Source: CAD feature listing. Evaluate the final solid. Frame: model axes, mm. A direction names the side the tool comes from. Give positions to 0.01 mm unless a question says otherwise; leave off trailing zeros. Order: outer loops, then holes, each group sorted by start corner. A loop starts at its lowest first (then second) coordinate and runs counter-clockwise, first axis right, second up. Notation, with made-up numbers: M -1,69 L 39,69 A14 ccw 39,76 Z; hole C 84,-11.5 d11. An arc over 180 degrees is marked long. Answer in a Markdown table with one row per item. Add a question column.
(1) Set-up query: faces 1 (the face through (-14.985, 0.66, 12.028)), 2 (the face through (4, 4, 4)), 3 (the face through (0, -2, 5)). Return all of +Z, -Z, +X, -X, +Y, -Y with unobstructed straight access to the full face (end or side cutting, diameter ignored); none if empty.
(2) Section query D-D, the plane y = 6. Return loops of the section in (x, z), plus the area to 3 significant figures.
(3) Mould query, pull axis Y, two halves, no side actions, for faces 4 (the face through (14.985, 0.66, 1.972)), 5 (the face through (2.2, 0.1, 0)), 6 (the face through (20.03, 6.31, 6.9)). Classes: pulls with the +Y half, pulls with the -Y half, needs draft (parallel to the pull), parting line crosses it, or undercut.
(4) Section query B-B, the plane y = 0. Return loops of the section in (x, z).
(5) Pin query (flat end, axial travel): P1, Ø3.5, axis at x = -10.39, y = -6, coming from the -Z side; P2, Ø5, axis at x = 16.5, z = 9.5, coming from the -Y side; P3, Ø4.5, axis at x = 10.39, y = -6, coming from the -Z side; P4, Ø8, axis at x = 11, z = 12, coming from the -Y side. Return the tip coordinate at first contact, or that it passes through.
(6) Section query A-A, the plane x = 0. Return loops of the section in (y, z).
(7) Material intervals for line 1 along Y through (x, z) = (0, 3.5); line 2 along Y through (x, z) = (0, 7.25); line 3 along X through (y, z) = (-6, 5.25), sorted ascending.
(8) Section query C-C, the plane z = 9.5. Return loops of the section in (x, y).
from build123d import *

# Parameters (mm, degrees)
SKETCH1_R           = 21
SKETCH1_R_2         = 2
BOSS_EXTRUDE1_DEPTH = 14
SKETCH2_R           = 15
CUT_EXTRUDE1_DEPTH  = 4
SKETCH3_R           = 15
SKETCH3_R_2         = 5
CUT_EXTRUDE2_DEPTH  = 4


with BuildPart() as part:
    # Sketch1 → Boss-Extrude1 (new body)
    with BuildSketch(Plane.XY):
        Circle(SKETCH1_R)
        with Locations((0, 12)):
            Circle(SKETCH1_R_2, mode=Mode.SUBTRACT)
        with Locations((10.392304845, 6)):
            Circle(SKETCH1_R_2, mode=Mode.SUBTRACT)
        with Locations((10.392304845, -6)):
            Circle(SKETCH1_R_2, mode=Mode.SUBTRACT)
        with Locations((0, -12)):
            Circle(SKETCH1_R_2, mode=Mode.SUBTRACT)
        with Locations((-10.392304845, -6)):
            Circle(SKETCH1_R_2, mode=Mode.SUBTRACT)
        with Locations((-10.392304845, 6)):
            Circle(SKETCH1_R_2, mode=Mode.SUBTRACT)
        Circle(SKETCH1_R_2, mode=Mode.SUBTRACT)
    extrude(amount=BOSS_EXTRUDE1_DEPTH)

    # Sketch2 → Cut-Extrude1 (cut)
    with BuildSketch(Plane.XY.offset(14)):
        Circle(SKETCH2_R)
    extrude(amount=-CUT_EXTRUDE1_DEPTH, mode=Mode.SUBTRACT)

    # Sketch3 → Cut-Extrude2 (cut)
    with BuildSketch(Plane(origin=(0, 0, 0), x_dir=(-1, 0, 0), z_dir=(0, 0, -1))):
        Circle(SKETCH3_R)
        Circle(SKETCH3_R_2, mode=Mode.SUBTRACT)
    extrude(amount=-CUT_EXTRUDE2_DEPTH, mode=Mode.SUBTRACT)


solid = part.part
Values follow:
| question | item | result |
|---|---|---|
| 1 | face 1 | +Z |
| 1 | face 2 | -Z |
| 1 | face 3 | +Z, -Z |
| 2 | outline | M -20.12,0 L -13.75,0 L -13.75,4 L -12.39,4 L -12.39,10 L -13.75,10 L -13.75,14 L -20.12,14 Z; M -8.39,4 L 8.39,4 L 8.39,10 L -8.39,10 Z; M 12.39,4 L 13.75,4 L 13.75,0 L 20.12,0 L 20.12,14 L 13.75,14 L 13.75,10 L 12.39,10 Z |
| 2 | area | 296 mm² |
| 3 | face 4 | undercut |
| 3 | face 5 | needs draft |
| 3 | face 6 | parting line crosses it |
| 4 | outline | M -21,0 L -15,0 L -15,4 L -5,4 L -5,0 L -2,0 L -2,10 L -15,10 L -15,14 L -21,14 Z; M 2,0 L 5,0 L 5,4 L 15,4 L 15,0 L 21,0 L 21,14 L 15,14 L 15,10 L 2,10 Z |
| 5 | P1 | passes through |
| 5 | P2 | stops at y = -15.65 |
| 5 | P3 | stops at z = 4 |
| 5 | P4 | stops at y = -19.8 |
| 6 | outline | M -21,0 L -15,0 L -15,4 L -14,4 L -14,10 L -15,10 L -15,14 L -21,14 Z; M -10,4 L -5,4 L -5,0 L -2,0 L -2,10 L -10,10 Z; M 2,0 L 5,0 L 5,4 L 10,4 L 10,10 L 2,10 Z; M 14,4 L 15,4 L 15,0 L 21,0 L 21,14 L 15,14 L 15,10 L 14,10 Z |
| 7 | line 1 | y = -21 to -15, -5 to -2, 2 to 5, 15 to 21 |
| 7 | line 2 | y = -21 to -14, -10 to -2, 2 to 10, 14 to 21 |
| 7 | line 3 | x = -20.12 to -12.39, -8.39 to 8.39, 12.39 to 20.12 |
| 8 | outline | C 0,0 d42; hole C -10.39,-6 d4; hole C -10.39,6 d4; hole C 0,-12 d4; hole C 0,0 d4; hole C 0,12 d4; hole C 10.39,-6 d4; hole C 10.39,6 d4 |
